Here's the drawing with two shaded views (mm, measured from the low corner). I have some questions. A direction names the side the tool comes from. Give positions to 0.01 mm unless a question says otherwise; leave off trailing zeros. Write each loop counter-clockwise with the first axis right and the second up, starting at its lowest first coordinate (ties: lowest second). Pieces come first, ordered by that corner, then holes.
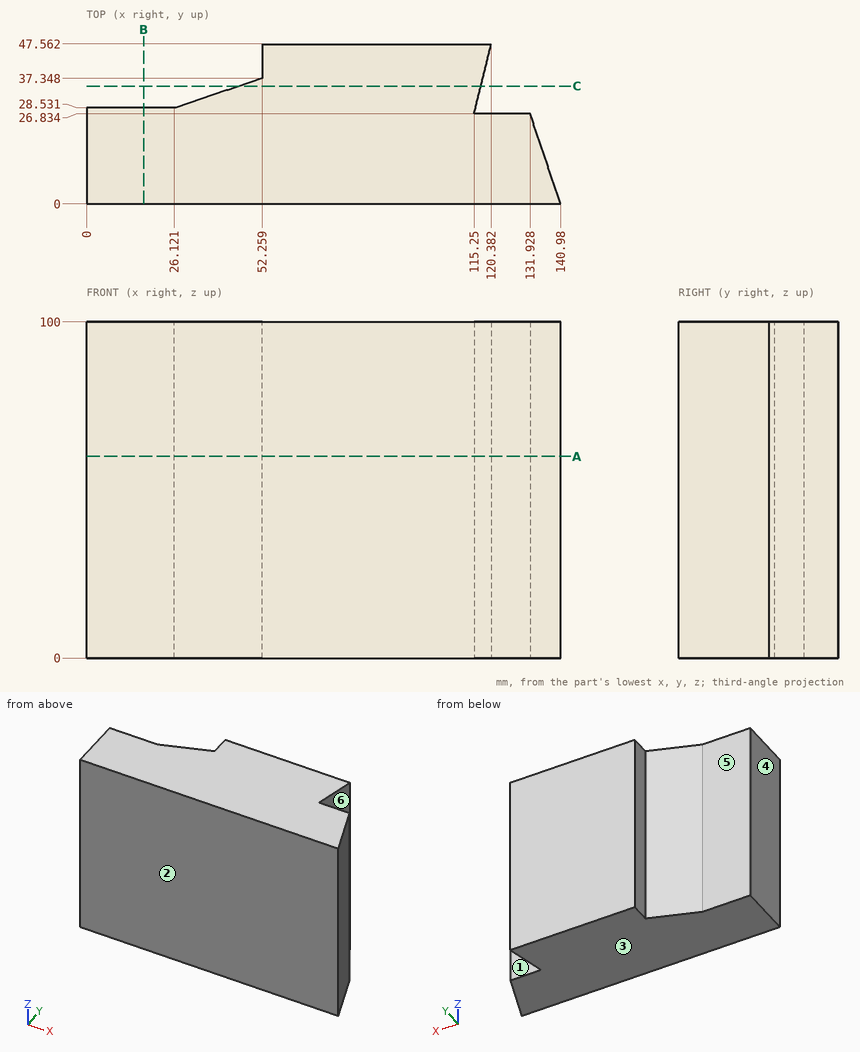
1) Suppose I cut it at B-B on x = 17. Write out the boundary of the cut face in (y, z), plus the area to 3 significant figures.
Values follow:
outline: (0, 0) - (28.53, 0) - (28.53, 100) - (0, 100) - close
area: 2,850 mm2
2) Suppose I cut it at A-A on z = 60. Write out the boundary of the cut face in (x, y), plus the area to 3 significant figures.
Values follow:
outline: (0, 0) - (140.98, 0) - (131.93, 26.83) - (115.25, 26.83) - (120.38, 47.56) - (52.26, 47.56) - (52.26, 37.35) - (26.12, 28.53) - (0, 28.53) - close
area: 5,220 mm2
3) Please list where these lines run through material, in increasing order: L1, parallel to Y at x = 7.5, z = 58; L2, parallel to X at y = 28, z = 47.5; L3, parallel to Y at x = 33, z = 54.5.
Values follow:
L1: y = 0 to 28.53
L2: x = 0 to 115.54
L3: y = 0 to 30.85
4) For pin 1 Ø13 at (x, z) = (15.5, 68.5) entering from +Y; pin 2 Ø1 at (y, z) = (8.5, 32.5) entering from +X, each with a flat end and sliding along its axis, tell me the tip position at first contact or that it passes through.
Values follow:
pin 1: stops at y = 28.53
pin 2: stops at x = 138.28
5) For the marked faces 4, 5 and 6, which set-ups out of +Z, -Z, +X, -X, +Y, -Y let a thin tool reach every point of the face, with its end or its side?
Values follow:
face 4: +Z, -Z, -X, +Y, -Y
face 5: +Z, -Z, -X, +Y
face 6: +Z, -Z, +X
6) Suppose I cut it at C-C on y = 35. Write out the boundary of the cut face in (x, z), plus the area to 3 significant figures.
Values follow:
outline: (45.3, 0) - (117.27, 0) - (117.27, 100) - (45.3, 100) - close
area: 7,200 mm2
7) If we mould it in two halves opening along Y, with no side actions, what happens to the marked faces 1, 2 and 3? For each: +Y half, -Y half, draft (parallel to the pull), parting line (faces both ways), or undercut.
Values follow:
face 1: undercut
face 2: -Y half
face 3: draft
